from build123d import *

# Parameters (mm, degrees)
SKETCH1_W           = 240
SKETCH1_H           = 120
BOSS_EXTRUDE1_DEPTH = 12
SKETCH2_R           = 32
CUT_EXTRUDE1_DEPTH  = 8
SKETCH3_W           = 23
SKETCH3_H           = 30.466372505
CUT_EXTRUDE2_DEPTH  = 8
SKETCH4_R           = 1.75
CUT_EXTRUDE4_DEPTH  = 20
SKETCH5_R           = 3
CUT_EXTRUDE7_DEPTH  = 5


with BuildPart() as part:
    # Sketch1 → Boss-Extrude1 (new body)
    with BuildSketch(Plane(origin=(0, 0, 0), x_dir=(1, 0, 0), z_dir=(0, 1, 0))):
        Rectangle(SKETCH1_W, SKETCH1_H)
    extrude(amount=-BOSS_EXTRUDE1_DEPTH)

    # Sketch2 → Cut-Extrude1 (cut)
    with BuildSketch(Plane(origin=(0, 0, 0), x_dir=(1, 0, 0), z_dir=(0, 1, 0))):
        with Locations(Location((0, 0, 0), (0, 0, 270))):
            Circle(SKETCH2_R)
    extrude(amount=-CUT_EXTRUDE1_DEPTH, mode=Mode.SUBTRACT)

    # Sketch3 → Cut-Extrude2 (cut)
    with BuildSketch(Plane(origin=(0, 0, 0), x_dir=(1, 0, 0), z_dir=(0, 1, 0))):
        with Locations((0, 44.766813748)):
            Rectangle(SKETCH3_W, SKETCH3_H)
    extrude(amount=-CUT_EXTRUDE2_DEPTH, mode=Mode.SUBTRACT)

    # Sketch4 → Cut-Extrude4 (cut)
    with BuildSketch(Plane(origin=(0, 0, 0), x_dir=(1, 0, 0), z_dir=(0, 1, 0))):
        with Locations(Location((-42.5, 0, 0), (0, 0, 270))):
            Circle(SKETCH4_R)
        with Locations(Location((-30.0520382, 30.0520382, 0), (0, 0, 270))):
            Circle(SKETCH4_R)
        with Locations(Location((30.0520382, 30.0520382, 0), (0, 0, 270))):
            Circle(SKETCH4_R)
        with Locations(Location((42.5, 0, 0), (0, 0, 270))):
            Circle(SKETCH4_R)
        with Locations(Location((30.0520382, -30.0520382, 0), (0, 0, 270))):
            Circle(SKETCH4_R)
        with Locations(Location((0, -42.5, 0), (0, 0, 270))):
            Circle(SKETCH4_R)
        with Locations(Location((-30.0520382, -30.0520382, 0), (0, 0, 270))):
            Circle(SKETCH4_R)
    extrude(amount=-CUT_EXTRUDE4_DEPTH, mode=Mode.SUBTRACT)

    # Sketch5 → Cut-Extrude7 (cut)
    with BuildSketch(Plane(origin=(0, -12, 0), x_dir=(1, 0, 0), z_dir=(0, 1, 0))):
        with Locations(Location((-42.5, 0, 0), (0, 0, 270))):
            Circle(SKETCH5_R)
        with Locations(Location((-30.0520382, 30.0520382, 0), (0, 0, 270))):
            Circle(SKETCH5_R)
        with Locations(Location((30.0520382, 30.0520382, 0), (0, 0, 270))):
            Circle(SKETCH5_R)
        with Locations(Location((42.5, 0, 0), (0, 0, 270))):
            Circle(SKETCH5_R)
        with Locations(Location((30.0520382, -30.0520382, 0), (0, 0, 270))):
            Circle(SKETCH5_R)
        with Locations(Location((0, -42.5, 0), (0, 0, 270))):
            Circle(SKETCH5_R)
        with Locations(Location((-30.0520382, -30.0520382, 0), (0, 0, 270))):
            Circle(SKETCH5_R)
    extrude(amount=CUT_EXTRUDE7_DEPTH, mode=Mode.SUBTRACT)


solid = part.part
For this review, take the finished solid that the model builds, in its own axes (mm). A direction names the side the tool comes from. Coordinates: 2 decimals unless noted, no trailing zeros. Order: outer loops, then holes, each group sorted by start corner. A loop starts at its lowest first (then second) coordinate and runs counter-clockwise, first axis right, second up. Notation, with made-up numbers: (-25.5, 67) - (-15.5, 67) arc R18 ccw to (-15.5, 91) - close; hole circle Ø3 at (65.5, 54.5). An arc over 180 degrees is marked (long way). Answer as CSV lines item,"result". Start each with the question number.
1) To check wall thickness, follow line 1 along X through (y, z) = (-8.2, 0); line 2 along X through (y, z) = (-2.5, 0); line 3 along X through (y, z) = (-9.75, -30). State the ranges of each line that lie inside material, in increasing order. Write a range as [from, to].
2) Machinability: for faces 5 (the cylindrical face through (27.123, -9.535, -30.702)), 6 (the flat face through (0, -8, -4)), 7 (the flat face through (-2, -6, 60)), 8 (the flat face through (-11.5, -4, -45)), which of the approach directions +Z, -Z, +X, -X, +Y, -Y give a long, thin tool a straight path to every point of the face, cutting with its end or side? Answer none if there is none.
3) Add section A-A (z = -43). State the section outline as (x, y) points, then the cut area to 3 significant figures.
4) Insertion check: P1, Ø1.8, axis at x = -30.5, z = -31, coming from the -Y side; P2, Ø3, axis at x = 42.5, z = 0, coming from the -Y side; P3, Ø8, axis at x = 8, z = 5, coming from the +Y side. Each pin has a flat end and moves straight along its axis. Give the tip position at first contact, or say it passes through.
5) Add section C-C (z = -22.5). State the section outline as (x, y) points, then the cut area to 3 significant figures.
6) Add section B-B (y = -4). State the section outline as (x, z) points.
7) Draft analysis for pull direction X (two halves, no side actions). For faces 1 (the flat face through (-30, -7, 32)), 2 (the flat face through (-28, 0, 26)), 3 (the flat face through (120, -6, 1)), 4 (the flat face through (-120, -6, 1)), state which applies: +X half, -X half, draft (parallel to the pull), parting line (faces both ways), or undercut.
Result:
1,line 1,"[-120, -45.5], [-39.5, 39.5], [45.5, 120]"
1,line 2,"[-120, -44.25], [-40.75, -32], [32, 40.75], [44.25, 120]"
1,line 3,"[-120, -33.05], [-27.05, 27.05], [33.05, 120]"
2,face 5,"-Y"
2,face 6,"+Y"
2,face 7,"+Z, +X, -X, +Y, -Y"
2,face 8,"-Z, +Y"
3,outline,"(-120, -12) - (120, -12) - (120, 0) - (11.5, 0) - (11.5, -8) - (-11.5, -8) - (-11.5, 0) - (-120, 0) - close"
3,area,"2,700 mm^2"
4,P1,"y = -7"
4,P2,"through"
4,P3,"y = -8"
5,outline,"(-120, -12) - (120, -12) - (120, 0) - (22.75, 0) - (22.75, -8) - (-22.75, -8) - (-22.75, 0) - (-120, 0) - close"
5,area,"2,520 mm^2"
6,outline,"(-120, -60) - (-11.5, -60) - (-11.5, -29.86) arc R32 cw (long way) to (11.5, -29.86) - (11.5, -60) - (120, -60) - (120, 60) - (-120, 60) - close; hole circle Ø3.5 at (-42.5, 0); hole circle Ø3.5 at (-30.05, -30.05); hole circle Ø3.5 at (-30.05, 30.05); hole circle Ø3.5 at (0, 42.5); hole circle Ø3.5 at (30.05, -30.05); hole circle Ø3.5 at (30.05, 30.05); hole circle Ø3.5 at (42.5, 0)"
7,face 1,"undercut"
7,face 2,"draft"
7,face 3,"+X half"
7,face 4,"-X half"
